```python
from build123d import *

# Parameters (mm, degrees)
SKETCH1_R           = 63.5
BOSS_EXTRUDE1_DEPTH = 12.7
SKETCH7_R           = 2.54
CUT_EXTRUDE2_DEPTH  = 91.696141042
CUT_EXTRUDE3_DEPTH  = 91.696141042


with BuildPart() as part:
    # Sketch1 → Boss-Extrude1 (new body)
    with BuildSketch(Plane(origin=(0, 0, 0), x_dir=(1, 0, 0), z_dir=(0, 1, 0))):
        with Locations(Location((0, 0, 0), (0, 0, 270))):
            Circle(SKETCH1_R)
    extrude(amount=-BOSS_EXTRUDE1_DEPTH)

    # Sketch7 → Cut-Extrude2 (cut, through all)
    with BuildSketch(Plane(origin=(0, 0, 0), x_dir=(1, 0, 0), z_dir=(0, 1, 0))):
        with Locations(Location((19.563011922, -13.687656502, 0), (0, 0, 270))):
            Circle(SKETCH7_R)
        with Locations(Location((21.635364211, 10.098237048, 0), (0, 0, 270))):
            Circle(SKETCH7_R)
        with Locations(Location((2.072352288, 23.78589355, 0), (0, 0, 270))):
            Circle(SKETCH7_R)
        with Locations(Location((-19.563011922, 13.687656502, 0), (0, 0, 270))):
            Circle(SKETCH7_R)
        with Locations(Location((-21.635364211, -10.098237048, 0), (0, 0, 270))):
            Circle(SKETCH7_R)
        with Locations(Location((-2.072352288, -23.78589355, 0), (0, 0, 270))):
            Circle(SKETCH7_R)
    extrude(amount=-CUT_EXTRUDE2_DEPTH, mode=Mode.SUBTRACT)

    # Sketch8 → Cut-Extrude3 (cut, through all)
    with BuildSketch(Plane(origin=(0, 0, 0), x_dir=(1, 0, 0), z_dir=(0, 1, 0))):
        Polygon((-5.623469851, -4.818771956), (1.361444003, -7.279453727), (6.984913855, -2.46068177), (5.623469851, 4.818771956), (-1.361444003, 7.279453727), (-6.984913855, 2.46068177), align=None)
    extrude(amount=-CUT_EXTRUDE3_DEPTH, mode=Mode.SUBTRACT)


solid = part.part
```
Check sheet for the modelled part. Datum: model origin and axes. Units: mm. A direction names the side the tool comes from. Coordinates: 2 decimals unless noted, no trailing zeros. Write each loop counter-clockwise with the first axis right and the second up, starting at its lowest first coordinate (ties: lowest second). Pieces come first, ordered by that corner, then holes. Notation, with made-up numbers: M 5,88.5 L 42,88.5 A12 cw 42,105.5 Z; hole C -8.5,74 d9. An arc over 180 degrees is marked long. Write item = value, one per line. Start each with the question number.
1. Sectioned sample at C-C (x = 53). Record the cut outline in (y, z) (3 decimals).
2. Sectioned sample at A-A (z = 0). Record the cut outline in (x, y), then the cut area to 3 significant figures.
3. Tool access check on faces 4 (the flat face through (-4.134, -6.261, -4.904)), 5 (the flat face through (-13, -12.7, -1)). Record the directions out of +Z, -Z, +X, -X, +Y, -Y that give a thin tool (end or side, any length) a straight path to the whole face; none if there is none.
4. Thickness scan on probe 1 along Z at (x, y) = (-3, -2.75); probe 2 along Z at (x, y) = (-2, -0.25); probe 3 along X at (y, z) = (-4.5, 13). Record the ranges inside material, lowest first.
5. Mould release check, pull along Z, two halves, no side actions. Record for faces 1 (the flat face through (-13, 0, -1)), 2 (the cylindrical face through (18.02, -6.26, 11.67)), 3 (the cylindrical face through (-61.99, -6.26, -13.77)): pulls with the +Z half, pulls with the -Z half, needs draft (parallel to the pull), parting line crosses it, or undercut.
6. Sectioned sample at B-B (y = -4). Record the cut outline in (x, z).
7. Go/stop test with flat-tipped pins: pin 1 (4 mm diameter, centred on y = -5.5, z = -7.5, fed in from +X); pin 2 (6 mm diameter, centred on x = -48.5, y = -2, fed in from +Z); pin 3 (6 mm diameter, centred on x = -7.5, y = -10, fed in from +Z); pin 4 (4 mm diameter, centred on x = -2.07, z = 23.79, fed in from -Y). Record where each tip stops, or that it passes through.
The answers:
q1.outline = M -12.7,-34.975 L 0,-34.975 L 0,34.975 L -12.7,34.975 Z
q2.outline = M -63.5,-12.7 L -6.52,-12.7 L -6.52,0 L -63.5,0 Z; M 6.52,-12.7 L 63.5,-12.7 L 63.5,0 L 6.52,0 Z
q2.area = 1,450 mm²
q3.face_4 = +Y, -Y
q3.face_5 = +Z, -Z, +X, -X, -Y
q4.probe_1 = -63.43 to -5.88, 5.74 to 21.42, 26.15 to 63.43
q4.probe_2 = -63.47 to -6.73, 6.1 to 21.25, 26.32 to 63.47
q4.probe_3 = -62.16 to 17.12, 22.01 to 62.16
q5.face_1 = needs draft
q5.face_2 = undercut
q5.face_3 = parting line crosses it
q6.outline = C 0,0 d127; hole C -21.64,10.1 d5.08; hole C -19.56,-13.69 d5.08; hole M -6.98,-2.46 L -1.36,-7.28 L 5.62,-4.82 L 6.98,2.46 L 1.36,7.28 L -5.62,4.82 Z; hole C -2.07,23.79 d5.08; hole C 2.07,-23.79 d5.08; hole C 19.56,13.69 d5.08; hole C 21.64,-10.1 d5.08
q7.pin_1 = 63.26
q7.pin_2 = 44.29
q7.pin_3 = 63.34
q7.pin_4 = through
